Build history of the part. All positions in model axes, mm. A direction names the side the tool comes from. Round coordinates to 2 decimals unless told otherwise and drop trailing zeros. Write each loop counter-clockwise with the first axis right and the second up, starting at its lowest first coordinate (ties: lowest second). Pieces come first, ordered by that corner, then holes.
1) Saw through at A-A (z = 12). Write the cut outline in (x, y), plus the area to 3 significant figures.
2) Saw through at B-B (x = -19). Write the cut outline in (y, z), plus the area to 3 significant figures.
3) Flat gauge pins, fed straight in: pin 1 (4 mm diameter, centred on x = 19, z = 13.5, fed in from +Y); pin 2 (4 mm diameter, centred on x = 24.5, y = 7, fed in from +Z); pin 3 (1.5 mm diameter, centred on y = -23.5, z = 13, fed in from -X). Where does each tip first touch, or does it go through?
4) Pull direction X, two halves, no side cores. Call faces 4 (the flat face through (-21.652, -20, 12)), 5 (the flat face through (38.348, -20, 12)), 6 (the cylindrical face through (-25.099, 8.436, 4.93)): +X half, -X half, draft (parallel to the pull), parting line (faces both ways), or undercut.
5) Which spindle directions (+Z, -Z, +X, -X, +Y, -Y) get a long thin tool onto all of the face, cutting with end or side? Do faces 1 (the flat face through (8, 0.127, 12)), 2 (the flat face through (8, -34.873, 12)), 3 (the flat face through (8, 17.627, 4)). Say none if no direction does.
6) Wall check: probe 1 along X at (y, z) = (-50, 4.5); probe 2 along Y at (x, z) = (6, 12.75); probe 3 along X at (y, z) = (-25, 12.75). Give the ranges that are in metal, low to high.
7) Saw through at D-D (x = -1.5). Write the cut outline in (y, z).
8) Saw through at C-C (y = -18.5). Write the cut outline in (x, z), plus the area to 3 significant figures.
from build123d import *

# Parameters (mm, degrees)
SKETCH_1_W      = 95.6
SKETCH_1_H      = 75
SKETCH_1_R      = 1.85
EXTRUDE_1_DEPTH = 10
FILLET_1_R      = 1.5
SKETCH_2_W      = 60
SKETCH_2_H      = 40
SKETCH_2_W_2    = 50
SKETCH_2_H_2    = 30
EXTRUDE_2_DEPTH = 5


with BuildPart() as part:
    # 草圖1 → 填料-伸長1 (new body)
    with BuildSketch(Plane.XY):
        with Locations((8.347810078, -19.873101952)):
            Rectangle(SKETCH_1_W, SKETCH_1_H)
        with Locations((-25.952189922, 10.076898048)):
            Circle(SKETCH_1_R, mode=Mode.SUBTRACT)
        with Locations((42.647810078, 10.076898048)):
            Circle(SKETCH_1_R, mode=Mode.SUBTRACT)
        with Locations((-25.952189922, -49.823101952)):
            Circle(SKETCH_1_R, mode=Mode.SUBTRACT)
        with Locations((42.647810078, -49.823101952)):
            Circle(SKETCH_1_R, mode=Mode.SUBTRACT)
    extrude(amount=EXTRUDE_1_DEPTH)

    # 圓角1
    fillet_1_edges = [part.edges().sort_by_distance(p)[0] for p in [
        (8.347810078, 17.626898048, 10),
        (8.347810078, -57.373101952, 10),
    ]]
    fillet(fillet_1_edges, radius=FILLET_1_R)

    # 草圖2 → 填料-伸長2 (add)
    with BuildSketch(Plane.XY.offset(10)):
        with Locations((8.347810078, -19.873101952)):
            Rectangle(SKETCH_2_W, SKETCH_2_H)
        with Locations((8.347810078, -19.873101952)):
            Rectangle(SKETCH_2_W_2, SKETCH_2_H_2, mode=Mode.SUBTRACT)
    extrude(amount=EXTRUDE_2_DEPTH)


solid = part.part
Evaluation:
1. outline: (-21.65, -39.87) - (38.35, -39.87) - (38.35, 0.13) - (-21.65, 0.13) - close; hole (-16.65, -34.87) - (33.35, -34.87) - (33.35, -4.87) - (-16.65, -4.87) - close
1. area: 900 mm2
2. outline: (-57.37, 0) - (17.63, 0) - (17.63, 8.5) arc R1.5 ccw to (16.13, 10) - (0.13, 10) - (0.13, 15) - (-39.87, 15) - (-39.87, 10) - (-55.87, 10) arc R1.5 ccw to (-57.37, 8.5) - close
2. area: 949 mm2
3. pin 1: stops at y = 0.13
3. pin 2: stops at z = 10
3. pin 3: stops at x = -21.65
4. face 4: -X half
4. face 5: +X half
4. face 6: undercut
5. face 1: +Z, +X, -X, +Y
5. face 2: +Z
5. face 3: +Z, -Z, +X, -X, +Y
6. probe 1: x = -39.45 to -27.79, -24.11 to 40.81, 44.49 to 56.15
6. probe 2: y = -39.87 to -34.87, -4.87 to 0.13
6. probe 3: x = -21.65 to -16.65, 33.35 to 38.35
7. outline: (-57.37, 0) - (17.63, 0) - (17.63, 8.5) arc R1.5 ccw to (16.13, 10) - (0.13, 10) - (0.13, 15) - (-4.87, 15) - (-4.87, 10) - (-34.87, 10) - (-34.87, 15) - (-39.87, 15) - (-39.87, 10) - (-55.87, 10) arc R1.5 ccw to (-57.37, 8.5) - close
8. outline: (-39.45, 0) - (56.15, 0) - (56.15, 10) - (38.35, 10) - (38.35, 15) - (33.35, 15) - (33.35, 10) - (-16.65, 10) - (-16.65, 15) - (-21.65, 15) - (-21.65, 10) - (-39.45, 10) - close
8. area: 1,010 mm2
